Can you work these out from the drawing? Everything is in mm from the part's minimum corner. A direction names the side the tool comes from. Round coordinates to 2 decimals unless told otherwise and drop trailing zeros. Write each loop counter-clockwise with the first axis right and the second up, starting at its lowest first coordinate (ties: lowest second). Pieces come first, ordered by that corner, then holes. Notation, with made-up numbers: (-6.5, 47) - (15.5, 47) arc R32 cw to (15.5, 81) - close; hole circle Ø11 at (87, 60). An arc over 180 degrees is marked (long way). One line per item, written item: value. Start each with the question number.
Item 1: Imagine slicing it at A-A, the plane z = 3. Please give me the cut outline in (x, y), then the cut area to 3 significant figures.
Item 2: Imagine slicing it at B-B, the plane x = 3. Please give me the cut outline in (y, z).
Item 3: For P1, Ø3, axis at x = 2, z = 3.5, coming from the -Y side; P2, Ø1.5, axis at x = 1.5, z = 1, coming from the +Y side, each with a flat end and sliding along its axis, tell me the tip position at first contact or that it passes through.
Item 4: For the marked faces 1 and 2, which set-ups out of +Z, -Z, +X, -X, +Y, -Y let a thin tool reach every point of the face, with its end or its side?
Item 5: If I drill on line 1 (Y direction, x = 4.3, z = 2.1); line 2 (Z direction, x = 2.95, y = 8.5); line 3 (Z direction, x = 1.5, y = 1.25), over which ranges is the centre line in solid material (lowest first)?
Item 6: Imagine slicing it at C-C, the plane y = 5.25. Please give me the cut outline in (x, z).
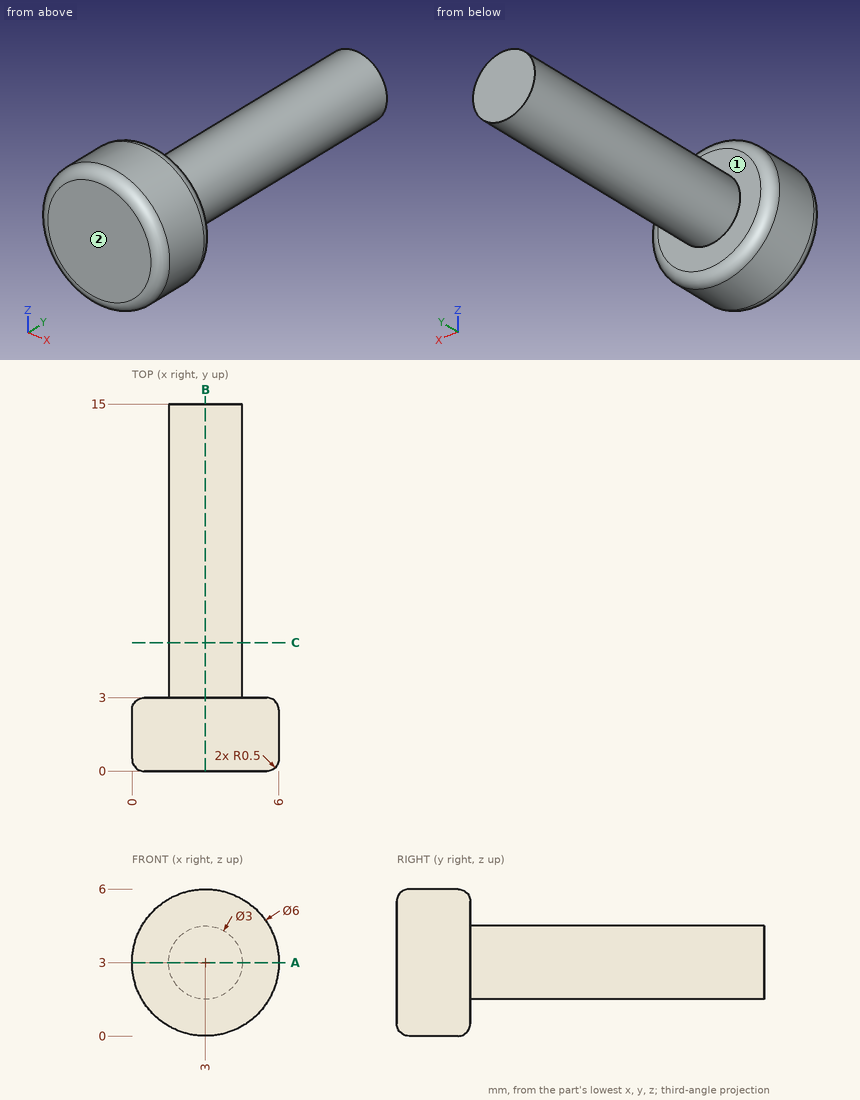
Values follow:
1. outline: (0, 0.5) arc R0.5 ccw to (0.5, 0) - (5.5, 0) arc R0.5 ccw to (6, 0.5) - (6, 2.5) arc R0.5 ccw to (5.5, 3) - (4.5, 3) - (4.5, 15) - (1.5, 15) - (1.5, 3) - (0.5, 3) arc R0.5 ccw to (0, 2.5) - close
1. area: 53.8 mm^2
2. outline: (0, 0.5) arc R0.5 ccw to (0.5, 0) - (2.5, 0) arc R0.5 ccw to (3, 0.5) - (3, 1.5) - (15, 1.5) - (15, 4.5) - (3, 4.5) - (3, 5.5) arc R0.5 ccw to (2.5, 6) - (0.5, 6) arc R0.5 ccw to (0, 5.5) - close
3. P1: stops at y = 0
3. P2: stops at y = 3
4. face 1: +Y
4. face 2: +Z, -Z, +X, -X, -Y
5. line 1: y = 0 to 3
5. line 2: z = 1.5 to 4.5
5. line 3: z = 0.4 to 5.6
6. outline: circle Ø3 at (3, 3)
